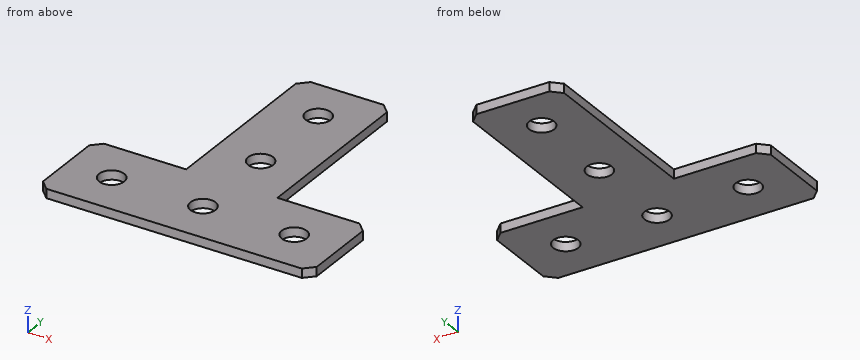
from build123d import *

# Parameters (mm, degrees)
EXTRUDE_1_DEPTH   = 2
HOLE_WIZARD_M51_D = 5.5
CHAMFER_1_SIZE    = 2


with BuildPart() as part:
    # Эскиз1 → Бобышка-Вытянуть1 (new body)
    with BuildSketch(Plane(origin=(0, 0, 0), x_dir=(1, 0, 0), z_dir=(0, 0, -1))):
        Polygon((-30, 60), (30, 60), (30, 40), (10, 40), (10, 0), (-10, 0), (-10, 40), (-30, 40), align=None)
    extrude(amount=EXTRUDE_1_DEPTH)

    # Отверстие с зазором M51 (through all)
    with Locations(Plane(origin=(0, 0, -2), x_dir=(1, 0, 0), z_dir=(0, 0, -1))):
        with Locations((0, 10), (0, 50), (-20, 50), (20, 50), (0, 30)):
            Hole(HOLE_WIZARD_M51_D / 2)

    # Фаска1
    chamfer_1_edges = [part.edges().sort_by_distance(p)[0] for p in [
        (-30, -40, -1),
        (-30, -60, -1),
        (30, -60, -1),
        (30, -40, -1),
        (10, 0, -1),
        (-10, 0, -1),
    ]]
    chamfer(chamfer_1_edges, length=CHAMFER_1_SIZE)


solid = part.part
Input: part model. Units: mm. Frame: model coordinates. Round coordinates to 2 decimals unless told otherwise and drop trailing zeros. Loops run counter-clockwise (first coordinate to the right, second up) from the corner with the lowest first, then second, coordinate; pieces in that order, holes last. Notation, with made-up numbers: M 56,45.25 L 113,45.25 A33 ccw 113,78.25 Z; hole C 46.5,26.5 d6. An arc over 180 degrees is marked long. Answer as CSV lines item,"result". Start each with the question number.
(1) Section A-A, the plane y = -10. Output: boundary loops of the cut face in (x, z).
(2) Section D-D, the plane y = -50. Output: boundary loops of the cut face in (x, z).
(3) Section B-B, the plane z = -0.9. Output: boundary loops of the cut face in (x, y).
(4) Line query: line 1 (X direction, y = -50, z = -0.6); line 2 (Y direction, x = 0, z = -0.6); line 3 (Y direction, x = 20, z = -0.7). Output: solid intervals per line, ascending. Write a range as [from, to].
(5) First-contact query: pin 1 (5 mm diameter, centred on x = 0, y = -10, fed in from +Z); pin 2 (0.6 mm diameter, centred on y = -30, z = -1.5, fed in from +X); pin 3 (1 mm diameter, centred on x = -17, z = -1, fed in from +Y). Flat tips, straight axial feed; report the tip coordinate or a pass-through.
(6) Section C-C, the plane x = 20. Output: boundary loops of the cut face in (y, z).
Values found:
1,outline,"M -10,-2 L -2.75,-2 L -2.75,0 L -10,0 Z; M 2.75,-2 L 10,-2 L 10,0 L 2.75,0 Z"
2,outline,"M -30,-2 L -22.75,-2 L -22.75,0 L -30,0 Z; M -17.25,-2 L -2.75,-2 L -2.75,0 L -17.25,0 Z; M 2.75,-2 L 17.25,-2 L 17.25,0 L 2.75,0 Z; M 22.75,-2 L 30,-2 L 30,0 L 22.75,0 Z"
3,outline,"M -30,-58 L -28,-60 L 28,-60 L 30,-58 L 30,-42 L 28,-40 L 10,-40 L 10,-2 L 8,0 L -8,0 L -10,-2 L -10,-40 L -28,-40 L -30,-42 Z; hole C -20,-50 d5.5; hole C 0,-50 d5.5; hole C 0,-30 d5.5; hole C 0,-10 d5.5; hole C 20,-50 d5.5"
4,line 1,"x = [-30, -22.75], [-17.25, -2.75], [2.75, 17.25], [22.75, 30]"
4,line 2,"y = [-60, -52.75], [-47.25, -32.75], [-27.25, -12.75], [-7.25, 0]"
4,line 3,"y = [-60, -52.75], [-47.25, -40]"
5,pin 1,"passes through"
5,pin 2,"stops at x = 10"
5,pin 3,"stops at y = -40"
6,outline,"M -60,-2 L -52.75,-2 L -52.75,0 L -60,0 Z; M -47.25,-2 L -40,-2 L -40,0 L -47.25,0 Z"
